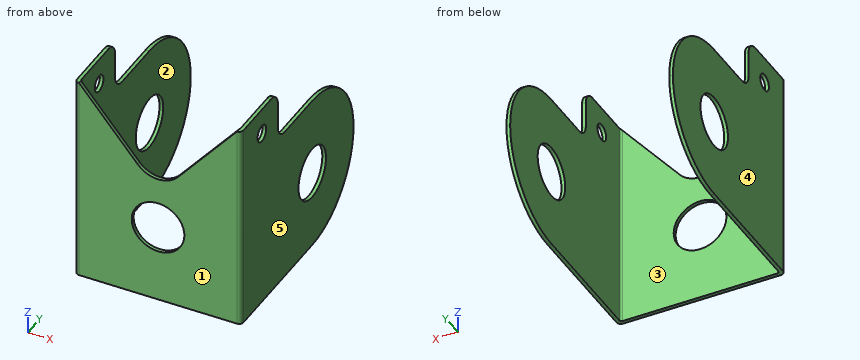
from build123d import *

# Parameters (mm, degrees)
F1_DEPTH = 50.8
F2_R     = 6.35
F3_DEPTH = 25.4
F4_R     = 6.35
F4_R_2   = 2
F5_DEPTH = 40.133


# Not quite as in the source:
# - a feature names something its author has since deleted; it is built from what else it names


with BuildPart() as f1:
    # F0 (on Top) → F1 (new body)
    with BuildSketch(Plane.XY):
        with BuildLine():
            Line((-39.116, 0), (-1.016, 0))
            ThreePointArc((-1.016, 0), (-0.2975795103, 0.2975795103), (0, 1.016))
            Line((0, 1.016), (0, 51.816))
            Line((0, 51.816), (-0.889, 51.816))
            Line((-0.889, 51.816), (-0.889, 1.397))
            ThreePointArc((-0.889, 1.397), (-1.0377897552, 1.0377897552), (-1.397, 0.889))
            Line((-1.397, 0.889), (-38.735, 0.889))
            ThreePointArc((-38.735, 0.889), (-39.0942102448, 1.0377897552), (-39.243, 1.397))
            Line((-39.243, 1.397), (-39.243, 51.816))
            Line((-39.243, 51.816), (-40.132, 51.816))
            Line((-40.132, 51.816), (-40.132, 1.016))
            ThreePointArc((-40.132, 1.016), (-39.8344204897, 0.2975795103), (-39.116, 0))
        make_face()
    extrude(amount=-F1_DEPTH)

    # F2 (on face) → F3 (cut)
    with BuildSketch(Plane.XZ):
        with Locations((-20.066, -31.75)):
            Circle(F2_R)
        with BuildLine():
            Line((-39.116, 0), (-24.915545424, -16.799318136))
            ThreePointArc((-24.915545424, -16.799318136), (-20.066, -19.05), (-15.216454576, -16.799318136))
            Line((-15.216454576, -16.799318136), (-1.016, 0))
            Line((-1.016, 0), (-39.116, 0))
        make_face()
    extrude(amount=-F3_DEPTH, mode=Mode.SUBTRACT)

    # F4 (on face) → F5 (cut, through all)
    with BuildSketch(Plane.YZ):
        with BuildLine():
            ThreePointArc((51.816, -31.75), (46.2363841816, -45.2203841816), (32.766, -50.8))
            Line((32.766, -50.8), (51.816, -50.8))
            Line((51.816, -50.8), (51.816, -31.75))
        make_face()
        with Locations((32.766, -31.75)):
            Circle(F4_R)
        with BuildLine():
            ThreePointArc((32.766, -12.7), (46.2363841816, -18.2796158184), (51.816, -31.75))
            Line((51.816, -31.75), (51.816, 0))
            Line((51.816, 0), (13.716, 0))
            ThreePointArc((13.716, 0), (15.9610640303, -0.9299359697), (16.891, -3.175))
            Line((16.891, -3.175), (16.891, -9.525))
            ThreePointArc((16.891, -9.525), (17.8209359697, -11.7700640303), (20.066, -12.7))
            Line((20.066, -12.7), (32.766, -12.7))
        make_face()
        with Locations((9.525, -6.35)):
            Circle(F4_R_2)
    extrude(amount=-F5_DEPTH, mode=Mode.SUBTRACT)


solid = f1.part
Design review of the part built by this model. Coordinates are the model's own, in mm. Face numbers are marked on the shaded views. A direction names the side the tool comes from. Coordinates: 2 decimals unless noted, no trailing zeros. Order: outer loops, then holes, each group sorted by start corner. A loop starts at its lowest first (then second) coordinate and runs counter-clockwise, first axis right, second up.
Item 1: For the marked faces 1 and 2, list the 3-axis set-ups (+Z, -Z, +X, -X, +Y, -Y) from which the entire face can be reached by the end or side of a thin tool; tool diameter is ignored.
Item 2: For pin 1 Ø5 at (x, z) = (-4, -30.5) entering from +Y, flat-tipped, find the tip position at first contact; note if it passes through.
Item 3: For line 1 (X direction, y = 3, z = -19); line 2 (Y direction, x = -11, z = -45); line 3 (Y direction, x = -39, z = -6), list the stretches that pass through material, from the lowest coordinate up.
Item 4: The part is to be moulded in two halves that separate along X. For the marked faces 3, 4 and 5, say which applies: pulls with the +X half, pulls with the -X half, needs draft (parallel to the pull), parting line crosses it, or undercut.
Item 5: Take a section at B-B, the plane y = 4. Write out the cut boundary in (x, z).
Item 6: Take a section at D-D, the plane z = -14. Write out the cut boundary in (x, y) (3 decimals).
Item 7: Take a section at A-A, the plane x = -20.5. Write out the cut boundary in (y, z), then the cut area to 3 significant figures.
Item 8: Take a section at C-C, the plane z = -6.35. Write out the cut boundary in (x, y) (3 decimals), then the cut area to 3 significant figures.
The answers:
1. face 1: +Z, -Z, +X, -X, -Y
1. face 2: +Z, -Z, +Y
2. pin 1: stops at y = 0.89
3. line 1: x = -40.13 to -39.24, -0.89 to 0
3. line 2: y = 0 to 0.89
3. line 3: y = 0 to 0.96
4. face 3: undercut
4. face 4: pulls with the -X half
4. face 5: pulls with the +X half
5. outline: (-40.13, -50.8) - (-39.24, -50.8) - (-39.24, 0) - (-40.13, 0) - close; (-0.89, -50.8) - (0, -50.8) - (0, 0) - (-0.89, 0) - close
6. outline: (-40.132, 1.016) arc R1.016 ccw to (-39.116, 0) - (-27.282, 0) - (-27.282, 0.889) - (-38.735, 0.889) arc R0.508 cw to (-39.243, 1.397) - (-39.243, 39.683) - (-40.132, 39.683) - close; (-12.85, 0) - (-1.016, 0) arc R1.016 ccw to (0, 1.016) - (0, 39.683) - (-0.889, 39.683) - (-0.889, 1.397) arc R0.508 cw to (-1.397, 0.889) - (-12.85, 0.889) - close
7. outline: (0, -50.8) - (0.89, -50.8) - (0.89, -38.09) - (0, -38.09) - close; (0, -25.41) - (0.89, -25.41) - (0.89, -19.04) - (0, -19.04) - close
7. area: 17.0 mm2
8. outline: (-40.132, 1.016) arc R1.016 ccw to (-39.116, 0) - (-33.748, 0) - (-33.748, 0.889) - (-38.735, 0.889) arc R0.508 cw to (-39.243, 1.397) - (-39.243, 7.525) - (-40.132, 7.525) - close; (-40.132, 11.525) - (-39.243, 11.525) - (-39.243, 16.891) - (-40.132, 16.891) - close; (-6.384, 0) - (-1.016, 0) arc R1.016 ccw to (0, 1.016) - (0, 7.525) - (-0.889, 7.525) - (-0.889, 1.397) arc R0.508 cw to (-1.397, 0.889) - (-6.384, 0.889) - close; (-0.889, 11.525) - (0, 11.525) - (0, 16.891) - (-0.889, 16.891) - close
8. area: 32.4 mm2
